Design review of the part built by this model. Coordinates are the model's own, in mm. A direction names the side the tool comes from. Give positions to 0.01 mm unless a question says otherwise; leave off trailing zeros. Loops run counter-clockwise (first coordinate to the right, second up) from the corner with the lowest first, then second, coordinate; pieces in that order, holes last.
from build123d import *

# Parameters (mm, degrees)
BOSS_EXTRUDE1_DEPTH = 26
FILLET1_R           = 6
FILLET2_R           = 4
BOSS_EXTRUDE2_DEPTH = 26
LPATTERN1_COUNT     = 6
LPATTERN1_PITCH     = 6
CUT_EXTRUDE1_DEPTH  = 145.300050087
CUT_EXTRUDE2_DEPTH  = 9
SKETCH5_R           = 1.5
CUT_EXTRUDE3_DEPTH  = 145.300050087
SKETCH6_R           = 1.75
BOSS_EXTRUDE4_DEPTH = 3
SKETCH7_R           = 1.55
CUT_EXTRUDE4_DEPTH  = 1
SKETCH8_R           = 1.55
CUT_EXTRUDE9_DEPTH  = 1


with BuildPart() as part:
    # Sketch1 → Boss-Extrude1 (new body)
    with BuildSketch(Plane(origin=(0, 0, 0), x_dir=(1, 0, 0), z_dir=(0, 1, 0))):
        with BuildLine():
            Line((-50.731616693, -70.850705373), (-59.243664017, -78.187515911))
            Line((-59.243664017, -78.187515911), (-62.093532673, -80.643910429))
            Line((-62.093532673, -80.643910429), (-63.59680926, -90.530272728))
            Line((-63.59680926, -90.530272728), (-50.927362258, -93.443194403))
            Line((-50.927362258, -93.443194403), (-33.202701652, -117.647252046))
            Line((-33.202701652, -117.647252046), (-33.202701652, -124.647252046))
            Line((-33.202701652, -124.647252046), (-22.202701652, -124.647252046))
            Line((-22.202701652, -124.647252046), (-22.202701652, -74.647252046))
            Line((-22.202701652, -74.647252046), (-15.131633841, -67.576184234))
            ThreePointArc((-15.131633841, -67.576184234), (-16.26454773, -59.166873554), (-24.673858411, -60.299787444))
            Line((-24.673858411, -60.299787444), (-27.876609184, -70.850705373))
            Line((-27.876609184, -70.850705373), (-50.731616693, -70.850705373))
        make_face()
        Polygon((-50.731616693, -70.850705373), (-59.243664017, -78.187515911), (-68.459423033, -8.796812025), (-46.129709685, 0), align=None)
    extrude(amount=BOSS_EXTRUDE1_DEPTH)

    # Fillet1
    fillet1_edges = [part.edges().sort_by_distance(p)[0] for p in [
        (-68.459423033, 13, 8.796812025),
        (-46.129709685, 13, 0),
    ]]
    fillet(fillet1_edges, radius=FILLET1_R)

    # Fillet2
    fillet2_edges = [part.edges().sort_by_distance(p)[0] for p in [
        (-33.202701652, 13, 124.647252046),
        (-63.59680926, 13, 90.530272728),
        (-62.093532673, 13, 80.643910429),
    ]]
    fillet(fillet2_edges, radius=FILLET2_R)

    # Sketch2 → Boss-Extrude2 (add)
    with BuildSketch(Plane(origin=(0, 26, 0), x_dir=(1, 0, 0), z_dir=(0, 1, 0))):
        Polygon((-22.202701652, -119.647252046), (-22.202701652, -121.647252046), (-18.202701652, -119.647252046), align=None)
        Polygon((-22.202701652, -117.647252046), (-22.202701652, -119.647252046), (-18.202701652, -119.647252046), align=None)
    boss_extrude2 = extrude(amount=-BOSS_EXTRUDE2_DEPTH)

    # LPattern1: Boss-Extrude2 ×6
    with Locations(*[(0, 0, -i * LPATTERN1_PITCH) for i in range(1, LPATTERN1_COUNT)]):
        add(boss_extrude2)

    # Sketch3 → Cut-Extrude1 (cut, through all)
    with BuildSketch(Plane(origin=(0, 26, 0), x_dir=(1, 0, 0), z_dir=(0, 1, 0))):
        Polygon((-25.014177768, -119.292756392), (-25.014177768, -94.292756392), (-40.014177768, -94.292756392), align=None)
    extrude(amount=-CUT_EXTRUDE1_DEPTH, mode=Mode.SUBTRACT)

    # Sketch4 → Cut-Extrude2 (cut)
    with BuildSketch(Plane(origin=(-77.692274337, 0, 56.894146205), x_dir=(0.5908220201984185, 0, 0.8068019214458154), z_dir=(-0.8068019214458154, 0, 0.5908220201984185))):
        Polygon((52.301141737, 23), (52.301141737, 4.095051152), (70.301141737, 8.273318832), (70.301141737, 19.575190426), align=None)
    extrude(amount=-CUT_EXTRUDE2_DEPTH, mode=Mode.SUBTRACT)

    # Sketch5 → Cut-Extrude3 (cut, through all)
    with BuildSketch(Plane(origin=(0, 26, 0), x_dir=(1, 0, 0), z_dir=(0, 1, 0))):
        with Locations(Location((-61.893792149, -12.659081905, 0), (0, 0, 270))):
            Circle(SKETCH5_R)
    extrude(amount=-CUT_EXTRUDE3_DEPTH, mode=Mode.SUBTRACT)

    # Sketch6 → Boss-Extrude4 (add)
    with BuildSketch(Plane(origin=(0, 26, 0), x_dir=(1, 0, 0), z_dir=(0, 1, 0))):
        with Locations(Location((-59.084491881, -87.463369105, 0), (0, 0, 270))):
            Circle(SKETCH6_R)
        with Locations(Location((-19.902746126, -63.937985839, 0), (0, 0, 270))):
            Circle(SKETCH6_R)
    extrude(amount=BOSS_EXTRUDE4_DEPTH)

    # Sketch7 → Cut-Extrude4 (cut)
    with BuildSketch(Plane(origin=(0, 29, 0), x_dir=(1, 0, 0), z_dir=(0, 1, 0))):
        with Locations(Location((-59.084491881, -87.463369105, 0), (0, 0, 270))):
            Circle(SKETCH7_R)
    extrude(amount=-CUT_EXTRUDE4_DEPTH, mode=Mode.SUBTRACT)

    # Sketch8 → Cut-Extrude9 (cut)
    with BuildSketch(Plane(origin=(0, 29, 0), x_dir=(1, 0, 0), z_dir=(0, 1, 0))):
        with Locations(Location((-19.902746126, -63.937985839, 0), (0, 0, 270))):
            Circle(SKETCH8_R)
    extrude(amount=-CUT_EXTRUDE9_DEPTH, mode=Mode.SUBTRACT)


solid = part.part
Q1. Insertion check: pin 1 (5 mm diameter, centred on y = 19, z = 35.5, fed in from +X); pin 2 (10 mm diameter, centred on y = 21, z = 27.5, fed in from +X); pin 3 (3 mm diameter, centred on x = -58.5, y = 26, fed in from -Z). Each pin has a flat end and moves straight along its axis. Give the tip position at first contact, or say it passes through.
Results:
pin 1: stops at x = -48.27
pin 2: stops at x = -47.59
pin 3: stops at z = 4.28
Q2. Take a section at C-C (z = 24.5). Give the boundary of the cut face in (x, y).
Results:
outline: (-66.37, 0) - (-47.72, 0) - (-47.72, 26) - (-66.37, 26) - close
Q3. Tool access review of faces 4 (the face through (-63.482, 12.818, 46.271)), 5 (the face through (-48.71, 12.82, 39.71)), 6 (the face through (-20.23, 13.18, 96.66)): name each direction out of +Z, -Z, +X, -X, +Y, -Y from which nothing blocks a thin tool from reaching the whole face with its end or side.
Results:
face 4: -X, +Y, -Y
face 5: +Y, -Y
face 6: +X, +Y, -Y
Q4. Draft analysis for pull direction X (two halves, no side actions). For faces 1 (the face through (-43.21, 13.68, 96.47)), 2 (the face through (-58.559, 27.479, 89.133)), 3 (the face through (-62.672, 12.818, 84.451)), state which applies: pulls with the +X half, pulls with the -X half, needs draft (parallel to the pull), parting line crosses it, or undercut.
Results:
face 1: undercut
face 2: parting line crosses it
face 3: pulls with the -X half
Q5. Take a section at A-A (y = 2). Give the number of separate pieces and of enclosed holes in the cut face, plus the area to 3 significant figures.
Results:
separate pieces: 1
enclosed holes: 2
area: 2,460 mm2
Q6. Wall thickness on line 1 (Y direction, x = -39, z = 77.5); line 2 (Z direction, x = -34.5, y = 14); line 3 (Z direction, x = -38.5, y = 9.75): over which ranges is each line inside the solid? List them lowest first.
Results:
line 1: y = 0 to 26
line 2: z = 70.85 to 94.29, 112.4 to 115.88
line 3: z = 70.85 to 94.29
Q7. Take a section at B-B (z = 44). Give the boundary of the cut face in (x, y).
Results:
outline: (-63.78, 0) - (-48.99, 0) - (-48.99, 26) - (-63.78, 26) - close
